The drawing under review shows one solid part. Ordinate dimensions are in mm from its lowest x, y, z. A direction names the side the tool comes from. Give positions to 0.01 mm unless a question says otherwise; leave off trailing zeros. Loops run counter-clockwise (first coordinate to the right, second up) from the corner with the lowest first, then second, coordinate; pieces in that order, holes last. Notation, with made-up numbers: M 72.25,25.25 L 116.25,25.25 A7 ccw 116.25,36.25 Z; hole C -6.5,-39 d7. An arc over 180 degrees is marked long. Answer as CSV lines item,"result".
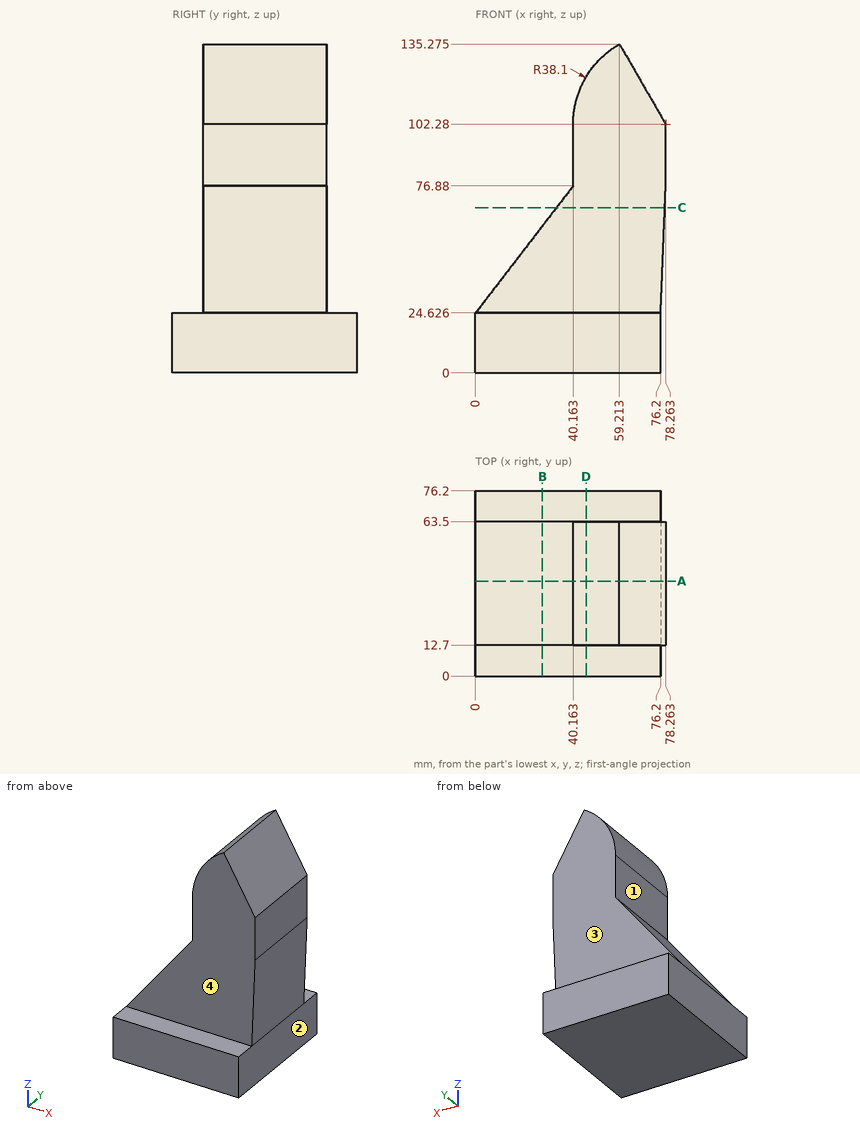
1. We need section D-D, the plane x = 45.5. Write out the cut boundary in (y, z) (1 decimal).
Answer block:
outline,"M 0,0 L 76.2,0 L 76.2,24.6 L 63.5,24.6 L 63.5,121.7 L 12.7,121.7 L 12.7,24.6 L 0,24.6 Z"
2. We need section A-A, the plane y = 39. Write out the cut boundary in (x, z) (1 decimal), plus the area to 3 significant figures.
Answer block:
outline,"M 0,0 L 76.2,0 L 76.2,24.6 L 78.3,76.9 L 78.3,102.3 L 59.2,135.3 A38.1 ccw 40.2,102.3 L 40.2,76.9 L 0,24.6 Z"
area,"6,590 mm²"
3. To check wall thickness, follow L1, parallel to X at y = 5, z = 11.5; L2, parallel to Z at x = 6, y = 65.5 (1 decimal); L3, parallel to Y at x = 48.5, z = 85. State the ranges of each line that lie inside material, in increasing order. Write a range as [from, to].
Answer block:
L1,"[0, 76.2]"
L2,"[0, 24.6]"
L3,"[12.7, 63.5]"
4. For the marked faces 1, 2, 3 and 4, list the 3-axis set-ups (+Z, -Z, +X, -X, +Y, -Y) from which the entire face can be reached by the end or side of a thin tool; tool diameter is ignored.
Answer block:
face 1,"+Z, -X, +Y, -Y"
face 2,"-Z, +X, +Y, -Y"
face 3,"+Z, +X, -X, +Y"
face 4,"+Z, +X, -X, -Y"
5. For P1, Ø5, axis at x = 42.5, y = 44, coming from the +Z side; P2, Ø7.5, axis at y = 36.5, z = 87, coming from the -X side; P3, Ø1, axis at x = 9.5, y = 28.5, coming from the +Z side (1 decimal); P4, Ø23.5, axis at x = 27.5, z = 86, coming from the -Y side, all flat-tipped, find the tip position at first contact; note any pin that passes through.
Answer block:
P1,"z = 120.86"
P2,"x = 40.16"
P3,"z = 37.6"
P4,"through"
6. We need section B-B, the plane x = 27.5. Write out the cut boundary in (y, z) (1 decimal), plus the area to 3 significant figures.
Answer block:
outline,"M 0,0 L 76.2,0 L 76.2,24.6 L 63.5,24.6 L 63.5,60.4 L 12.7,60.4 L 12.7,24.6 L 0,24.6 Z"
area,"3,690 mm²"
7. We need section C-C, the plane z = 68. Write out the cut boundary in (x, y), plus the area to 3 significant figures.
Answer block:
outline,"M 33.34,12.7 L 77.91,12.7 L 77.91,63.5 L 33.34,63.5 Z"
area,"2,260 mm²"
